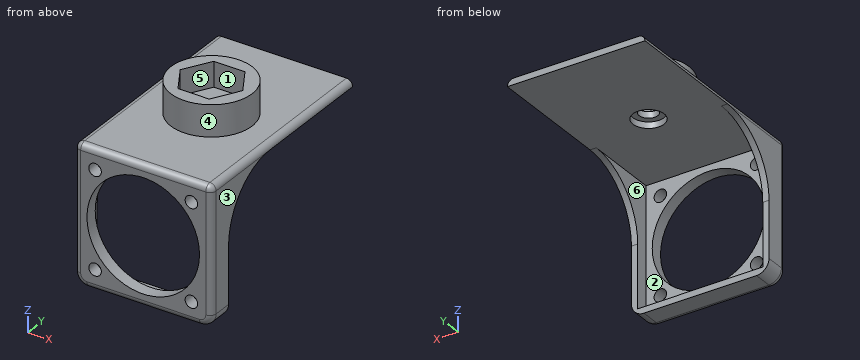
```python
from build123d import *

# Parameters (mm, degrees)
SKETCH_1_W          = 22
SKETCH_1_H          = 22
SKETCH_1_W_2        = 20
SKETCH_1_H_2        = 20
EXTRUDE_1_DEPTH     = 4
SKETCH_2_W          = 20
SKETCH_2_H          = 20
EXTRUDE_2_DEPTH     = 2
CUT_EXTRUDE_1_DEPTH = 2
SKETCH_4_R          = 1
CUT_EXTRUDE_2_DEPTH = 2
EXTRUDE_4_DEPTH     = 30
CUT_EXTRUDE_3_DEPTH = 46.617978912
SKETCH_8_R          = 2.5
CUT_EXTRUDE_4_DEPTH = 4
SKETCH_10_R         = 6.5
EXTRUDE_5_DEPTH     = 5
CUT_EXTRUDE_5_DEPTH = 4
SKETCH_12_R         = 1.5
CUT_EXTRUDE_6_DEPTH = 4
FILLET_2_R          = 2
FILLET_3_R          = 2
FILLET_4_R          = 1
FILLET_5_R          = 1
FILLET_6_R          = 1


with BuildPart() as part:
    # 草图1 → 凸台-拉伸1 (new body)
    with BuildSketch(Plane(origin=(0, 0, 0), x_dir=(1, 0, 0), z_dir=(0, 1, 0))):
        with Locations((10, 10)):
            Rectangle(SKETCH_1_W, SKETCH_1_H)
        with Locations((10, 10)):
            Rectangle(SKETCH_1_W_2, SKETCH_1_H_2, mode=Mode.SUBTRACT)
    extrude(amount=EXTRUDE_1_DEPTH)

    # 草图2 → 凸台-拉伸2 (add)
    with BuildSketch(Plane(origin=(0, 0, 0), x_dir=(1, 0, 0), z_dir=(0, 1, 0))):
        with Locations((10, 10)):
            Rectangle(SKETCH_2_W, SKETCH_2_H)
    extrude(amount=EXTRUDE_2_DEPTH)

    # 草图3 → 切除-拉伸1 (cut)
    with BuildSketch(Plane(origin=(0, 2, 0), x_dir=(1, 0, 0), z_dir=(0, 1, 0))):
        with BuildLine():
            ThreePointArc((19, 10), (10, 19), (1, 10))
            Line((1, 10), (19, 10))
        make_face()
        with BuildLine():
            Line((19, 10), (1, 10))
            ThreePointArc((1, 10), (10, 1), (19, 10))
        make_face()
    extrude(amount=-CUT_EXTRUDE_1_DEPTH, mode=Mode.SUBTRACT)

    # 草图4 → 切除-拉伸2 (cut)
    with BuildSketch(Plane(origin=(0, 2, 0), x_dir=(1, 0, 0), z_dir=(0, 1, 0))):
        with Locations(Location((2.3, 17.7, 0), (0, 0, 270))):
            Circle(SKETCH_4_R)
        with Locations(Location((17.7, 17.7, 0), (0, 0, 270))):
            Circle(SKETCH_4_R)
        with Locations(Location((17.7, 2.3, 0), (0, 0, 270))):
            Circle(SKETCH_4_R)
        with Locations(Location((2.3, 2.3, 0), (0, 0, 270))):
            Circle(SKETCH_4_R)
    extrude(amount=-CUT_EXTRUDE_2_DEPTH, mode=Mode.SUBTRACT)

    # 草图5 → 凸台-拉伸4 (add)
    with BuildSketch(Plane(origin=(0, 4, 0), x_dir=(1, 0, 0), z_dir=(0, 1, 0))):
        Polygon((0, 0), (0, 10), (-1, 10), (-1, -1), (21, -1), (21, 10), (20, 10), (20, 0), align=None)
    extrude(amount=EXTRUDE_4_DEPTH)

    # 草图7 → 切除-拉伸3 (cut, through all)
    with BuildSketch(Plane.ZY.offset(1)):
        with BuildLine():
            ThreePointArc((-10, 4), (-2.928932188, 6.928932188), (0, 14))
            Line((0, 14), (-10, 14))
            Line((-10, 14), (-10, 4))
        make_face()
        with BuildLine():
            Line((-10, 14), (0, 14))
            ThreePointArc((0, 14), (-2.928932188, 21.071067812), (-10, 24))
            Line((-10, 24), (-10, 14))
        make_face()
        with BuildLine():
            Line((0, 14), (0, 34))
            Line((0, 34), (-10, 34))
            Line((-10, 34), (-10, 24))
            ThreePointArc((-10, 24), (-2.928932188, 21.071067812), (0, 14))
        make_face()
    extrude(amount=-CUT_EXTRUDE_3_DEPTH, mode=Mode.SUBTRACT)

    # 草图8 → 切除-拉伸4 (cut)
    with BuildSketch(Plane(origin=(0, 0, 0), x_dir=(-1, 0, 0), z_dir=(0, 0, -1))):
        with Locations((-10, 16.5)):
            Circle(SKETCH_8_R)
    extrude(amount=-CUT_EXTRUDE_4_DEPTH, mode=Mode.SUBTRACT)

    # 草图10 → 凸台-拉伸5 (add)
    with BuildSketch(Plane.XY.offset(1)):
        with Locations(Location((10, 16.5, 0), (0, 0, 180))):
            Circle(SKETCH_10_R)
    extrude(amount=EXTRUDE_5_DEPTH)

    # 草图11 → 切除-拉伸5 (cut)
    with BuildSketch(Plane.XY.offset(6)):
        Polygon((15, 16.5), (12.5, 20.830127019), (7.5, 20.830127019), (5, 16.5), (7.5, 12.169872981), (12.5, 12.169872981), align=None)
    extrude(amount=-CUT_EXTRUDE_5_DEPTH, mode=Mode.SUBTRACT)

    # 草图12 → 切除-拉伸6 (cut)
    with BuildSketch(Plane(origin=(0, 0, 1), x_dir=(-1, 0, 0), z_dir=(0, 0, -1))):
        with Locations((-10, 16.5)):
            Circle(SKETCH_12_R)
    extrude(amount=-CUT_EXTRUDE_6_DEPTH, mode=Mode.SUBTRACT)

    # 圆角2
    fillet_2_edges = [part.edges().sort_by_distance(p)[0] for p in [
        (-1, 2, -21),
    ]]
    fillet(fillet_2_edges, radius=FILLET_2_R)

    # 圆角3
    fillet_3_edges = [part.edges().sort_by_distance(p)[0] for p in [
        (21, 2, -21),
    ]]
    fillet(fillet_3_edges, radius=FILLET_3_R)

    # 圆角4
    fillet_4_edges = [part.edges().sort_by_distance(p)[0] for p in [
        (21, 17, 1),
    ]]
    fillet(fillet_4_edges, radius=FILLET_4_R - 0.0001)  # a hair under: the kernel refuses the full size

    # 圆角5
    fillet_5_edges = [part.edges().sort_by_distance(p)[0] for p in [
        (-1, 17, 1),
    ]]
    fillet(fillet_5_edges, radius=FILLET_5_R - 0.0001)  # a hair under: the kernel refuses the full size

    # 圆角6
    fillet_6_edges = [part.edges().sort_by_distance(p)[0] for p in [
        (-1, 0, -9.49995),
        (-0.414213562, 0, -20.414213562),
        (10, 0, -21),
        (20.414213562, 0, -20.414213562),
        (21, 0, -9.49995),
        (20.707136071, 0, 0.707136071),
        (10, 0, 1),
        (-0.707136071, 0, 0.707136071),
    ]]
    fillet(fillet_6_edges, radius=FILLET_6_R - 0.0001)  # a hair under: the kernel refuses the full size


solid = part.part
```
Here's how the part is built. I have some questions about the finished solid (model axes, mm). Face numbers are marked on the shaded views. A direction names the side the tool comes from. Coordinates: 2 decimals unless noted, no trailing zeros. Order: outer loops, then holes, each group sorted by start corner. A loop starts at its lowest first (then second) coordinate and runs counter-clockwise, first axis right, second up.
1) Imagine slicing it at A-A on x = 10. State how many separate pieces and enclosed holes the cut face has, and give its area (3 significant figures).
2) Imagine slicing it at C-C on x = 4. List the corners of the cut face in (y, z) for me, and give its area (3 significant figures).
3) Will these pins go through, and if not, where does the flat tip stop? pin 1 (5 mm diameter, centred on x = 11, y = 6.5, fed in from +Z); pin 2 (12 mm diameter, centred on x = 6, z = -14.5, fed in from +Y); pin 3 (4.5 mm diameter, centred on x = 10, z = 3.5, fed in from -Y).
4) We'd pull the mould along Y, two halves only. Please class the marked faces 4, 5 and 6: +Y half, -Y half, draft (parallel to the pull), parting line (faces both ways), or undercut.
5) Imagine slicing it at D-D on x = 17.7. List the corners of the cut face in (y, z) for me.
6) Imagine slicing it at B-B on z = -8.5. List the corners of the cut face in (x, y) for me.
7) I need wall thicknesses on line 1 (Y direction, x = 10, z = 1.65); line 2 (X direction, y = 1, z = -2.3); line 3 (X direction, y = 3, z = -14.25). Which ranges of each line are inside material? Lowest first, please.
8) Which directions (+Z, -Z, +X, -X, +Y, -Y) give clear straight access to the entire face, cutting with the end or side of a thin tool? Please do the marked faces 1, 2 and 3.
Response values:
1. separate pieces: 3
1. enclosed holes: 0
1. area: 63.9 mm2
2. outline: (0, -20) arc R1 ccw to (1, -21) - (4, -21) - (4, -20) - (2, -20) - (2, -16.71) - (0, -16.71) - close; (0, -3.29) - (2, -3.29) - (2, 0) - (34, 0) - (34, 1) - (19, 1) - (19, 6) - (14, 6) - (14, 1) - (1, 1) arc R1 ccw to (0, 0) - close
2. area: 75.7 mm2
3. pin 1: stops at z = 1
3. pin 2: stops at y = 4
3. pin 3: stops at y = 10
4. face 4: parting line
4. face 5: undercut
4. face 6: draft
5. outline: (0, -20) arc R1 ccw to (1, -21) - (4, -21) - (4, -20) - (2, -20) - (2, -18.7) - (0, -18.7) - close; (0, -16.7) - (2, -16.7) - (2, -14.66) - (0, -14.66) - close; (0, -5.34) - (2, -5.34) - (2, -3.3) - (0, -3.3) - close; (0, -1.3) - (2, -1.3) - (2, 0) - (34, 0) - (34, 1) - (1, 1) arc R1 ccw to (0, 0) - close
6. outline: (-1, 1) arc R1 ccw to (0, 0) - (1.13, 0) - (1.13, 2) - (0, 2) - (0, 4.11) - (-1, 4.11) - close; (18.87, 0) - (20, 0) arc R1 ccw to (21, 1) - (21, 4.11) - (20, 4.11) - (20, 2) - (18.87, 2) - close
7. line 1: y = 10 to 15, 18 to 23
7. line 2: x = -1 to 1.3, 3.3 to 5.34, 14.66 to 16.7, 18.7 to 21
7. line 3: x = -1 to 0, 20 to 21
8. face 1: +Z
8. face 2: +Y
8. face 3: +Z, -Z, +X, +Y, -Y
